For this review, take the finished solid that the model builds, in its own axes (mm). A direction names the side the tool comes from. Give positions to 0.01 mm unless a question says otherwise; leave off trailing zeros. Write each loop counter-clockwise with the first axis right and the second up, starting at its lowest first coordinate (ties: lowest second). Pieces come first, ordered by that corner, then holes.
Q1. Machinability: for faces 4 (the flat face through (54, 0.686, 0)), 5 (the cylindrical face through (-65.77, 11.806, 10.41)), 6 (the flat face through (-0.889, 7.453, 11.29)), 7 (the flat face through (0.89, 32.31, -2.9)), 8 (the cylindrical face through (-68.039, 9.055, 10.25)), which of the approach directions +Z, -Z, +X, -X, +Y, -Y give a long, thin tool a straight path to every point of the face, cutting with its end or side? Answer none if there is none.
Q2. We need section A-A (y = 2). Give the number of separate pieces and of enclosed holes in the cut face, then the cut area to 3 significant figures.
Q3. For line 1 (X direction, y = 0.4, z = 0); line 2 (X direction, y = 6.5, z = 0); line 3 (X direction, y = 18, z = 4.5) (3 decimals), list the stretches that pass through material, from the lowest coordinate up.
Q4. Insertion check: P1, Ø6.5, axis at x = 50.8, z = 0, coming from the +Y side; P2, Ø4.5, axis at x = 50.5, z = 0, coming from the -Y side; P3, Ø3, axis at x = 16, y = 7, coming from the +Z side. Each pin has a flat end and moves straight along its axis. Give the tip position at first contact, or say it passes through.
Q5. Mouldability with a two-part tool opening along X and no side actions: class faces 1 (the flat face through (54, 0, -3)), 2 (the cylindrical face through (68, 32.5, -5)), 3 (the flat face through (-51, 10.16, 0)) as released by +X, released by -X, zero draft, split by the parting line, or undercut.
Q6. We need section B-B (x = 43). Write out the cut boundary in (y, z), then the cut area to 3 significant figures.
```python
from build123d import *

# Parameters (mm, degrees)
SKETCH2_R             = 6.35
BOSS_EXTRUDE1_DEPTH   = 19.05
BOSS_EXTRUDE1_2_DEPTH = 19.05
BOSS_EXTRUDE2_DEPTH   = 6.35
BOSS_EXTRUDE3_REACH   = 75.737
CUT_EXTRUDE1_DEPTH    = 3.175
CHAMFER2_SIZE         = 1.5875
HOLE1_D               = 5.715
HOLE1_DEPTH           = 10.16
HOLE1_CBORE_D         = 6.985
HOLE1_CBORE_DEPTH     = 0.6858


with BuildPart() as part:
    # Sketch2 → Boss-Extrude1 (new body)
    with BuildSketch(Plane(origin=(0, 0, 0), x_dir=(1, 0, 0), z_dir=(0, 1, 0))):
        with Locations(Location((-50.8, 0, 0), (0, 0, 90))):
            Circle(SKETCH2_R)
    extrude(amount=BOSS_EXTRUDE1_DEPTH)



with BuildPart() as body_2:
    # Sketch2 → Boss-Extrude1 2 (new body)
    with BuildSketch(Plane(origin=(0, 0, 0), x_dir=(1, 0, 0), z_dir=(0, 1, 0))):
        with Locations(Location((50.8, 0, 0), (0, 0, 90))):
            Circle(SKETCH2_R)
    extrude(amount=BOSS_EXTRUDE1_2_DEPTH)


with BuildPart() as part_1:
    add(part.part)

    add(body_2.part)  # Boss-Extrude2 merges body 2
    # Sketch3 → Boss-Extrude2 (add)
    with BuildSketch(Plane(origin=(0, 5.650833475, 8.701520484), x_dir=(-1, 0, 0), z_dir=(0, 0.5446390350150281, 0.8386705679454234))):
        with BuildLine():
            Line((-63.5, -31.851674319), (63.5, -31.851674319))
            ThreePointArc((63.5, -31.851674319), (67.990128061, -29.99180238), (69.85, -25.501674319))
            Line((69.85, -25.501674319), (69.85, -6.451674319))
            ThreePointArc((69.85, -6.451674319), (67.990128061, -1.961546259), (63.5, -0.101674319))
            Line((63.5, -0.101674319), (-63.5, -0.101674319))
            ThreePointArc((-63.5, -0.101674319), (-67.990128061, -1.961546259), (-69.85, -6.451674319))
            Line((-69.85, -6.451674319), (-69.85, -25.501674319))
            ThreePointArc((-69.85, -25.501674319), (-67.990128061, -29.99180238), (-63.5, -31.851674319))
        make_face()
    extrude(amount=BOSS_EXTRUDE2_DEPTH)

    # Sketch8 → Boss-Extrude3 (add, up to next)
    with BuildSketch(Plane(origin=(0, 19.05, 0), x_dir=(1, 0, 0), z_dir=(0, 1, 0)), mode=Mode.PRIVATE) as boss_extrude3_sk1:
        with BuildLine():
            Line((44.45, 0), (57.15, 0))
            ThreePointArc((57.15, 0), (50.8, 6.35), (44.45, 0))
        make_face()
    boss_extrude3_tool1 = extrude(boss_extrude3_sk1.sketch, amount=BOSS_EXTRUDE3_REACH, mode=Mode.PRIVATE) - part_1.part
    # Sketch8 → Boss-Extrude3 (add, up to next)
    with BuildSketch(Plane(origin=(0, 19.05, 0), x_dir=(1, 0, 0), z_dir=(0, 1, 0)), mode=Mode.PRIVATE) as boss_extrude3_sk2:
        with BuildLine():
            ThreePointArc((-44.45, 0), (-50.8, 6.35), (-57.15, 0))
            Line((-57.15, 0), (-44.45, 0))
        make_face()
    boss_extrude3_tool2 = extrude(boss_extrude3_sk2.sketch, amount=BOSS_EXTRUDE3_REACH, mode=Mode.PRIVATE) - part_1.part
    add(boss_extrude3_tool1.solids().sort_by_distance((50.8, 19.05, -2.695024))[0])
    add(boss_extrude3_tool2.solids().sort_by_distance((-50.8, 19.05, -2.695024))[0])

    # Sketch9 → Cut-Extrude1 (cut)
    with BuildSketch(Plane(origin=(0, 9.109291347, 14.02707859), x_dir=(1, 0, 0), z_dir=(0, 0.5446390350150282, 0.8386705679454234))):
        with BuildLine():
            Line((63.5, 28.676674319), (-63.5, 28.676674319))
            ThreePointArc((-63.5, 28.676674319), (-65.74506403, 27.74673835), (-66.675, 25.501674319))
            Line((-66.675, 25.501674319), (-66.675, 6.451674319))
            ThreePointArc((-66.675, 6.451674319), (-65.74506403, 4.206610289), (-63.5, 3.276674319))
            Line((-63.5, 3.276674319), (63.5, 3.276674319))
            ThreePointArc((63.5, 3.276674319), (65.74506403, 4.206610289), (66.675, 6.451674319))
            Line((66.675, 6.451674319), (66.675, 25.501674319))
            ThreePointArc((66.675, 25.501674319), (65.74506403, 27.74673835), (63.5, 28.676674319))
        make_face()
    extrude(amount=-CUT_EXTRUDE1_DEPTH, mode=Mode.SUBTRACT)

    # Chamfer2
    chamfer2_edges = [part_1.edges().sort_by_distance(p)[0] for p in [
        (67.990128061, 7.29592459, 7.633185823),
        (0, 5.736104734, 8.646144681),
        (-67.990128061, 7.29592459, 7.633185823),
        (67.990128061, 30.80407541, -7.633185823),
        (69.85, 19.05, 0),
        (67.990128061, 10.754382462, 12.958743929),
        (69.85, 22.508457872, 5.325558106),
        (67.990128061, 34.262533283, -2.307627716),
        (0, 32.363895266, -8.646144681),
        (-67.990128061, 30.80407541, -7.633185823),
        (-69.85, 19.05, 0),
        (-67.990128061, 10.754382462, 12.958743929),
        (0, 9.194562606, 13.971702787),
        (0, 35.822353138, -3.320586574),
        (-67.990128061, 34.262533283, -2.307627716),
        (-69.85, 22.508457872, 5.325558106),
    ]]
    chamfer(chamfer2_edges, length=CHAMFER2_SIZE)

    # Hole1
    with Locations(Plane(origin=(-50.8, 0, 0), x_dir=(0, 0, -1), z_dir=(0, -1, 0))):
        with Locations((0, 0), (0, 101.6)):
            CounterBoreHole(HOLE1_D / 2, HOLE1_CBORE_D / 2, HOLE1_CBORE_DEPTH, depth=HOLE1_DEPTH)


solid = part_1.part
```
Computed:
1. face 4: -Y
1. face 5: +Y
1. face 6: +Z, +X, -X, -Y
1. face 7: +Z
1. face 8: +Z, -X, -Y
2. separate pieces: 2
2. enclosed holes: 2
2. area: 202 mm2
3. line 1: x = -57.15 to -54.29, -47.31 to -44.45, 44.45 to 47.31, 54.29 to 57.15
3. line 2: x = -57.15 to -53.66, -47.94 to -44.45, 44.45 to 47.94, 53.66 to 57.15
3. line 3: x = -69.85 to -66.675, 66.675 to 69.85
4. P1: stops at y = 34.66
4. P2: stops at y = 10.16
4. P3: stops at z = 12.68
5. face 1: zero draft
5. face 2: released by +X
5. face 3: undercut
6. outline: (6.6, 9.98) - (7.07, 7.78) - (31.03, -7.78) - (33.23, -7.31) - (34.96, -4.65) - (34.49, -2.46) - (33.16, -1.59) - (31.43, -4.25) - (10.13, 9.58) - (11.86, 12.24) - (10.53, 13.11) - (8.33, 12.64) - close
6. area: 116 mm2
